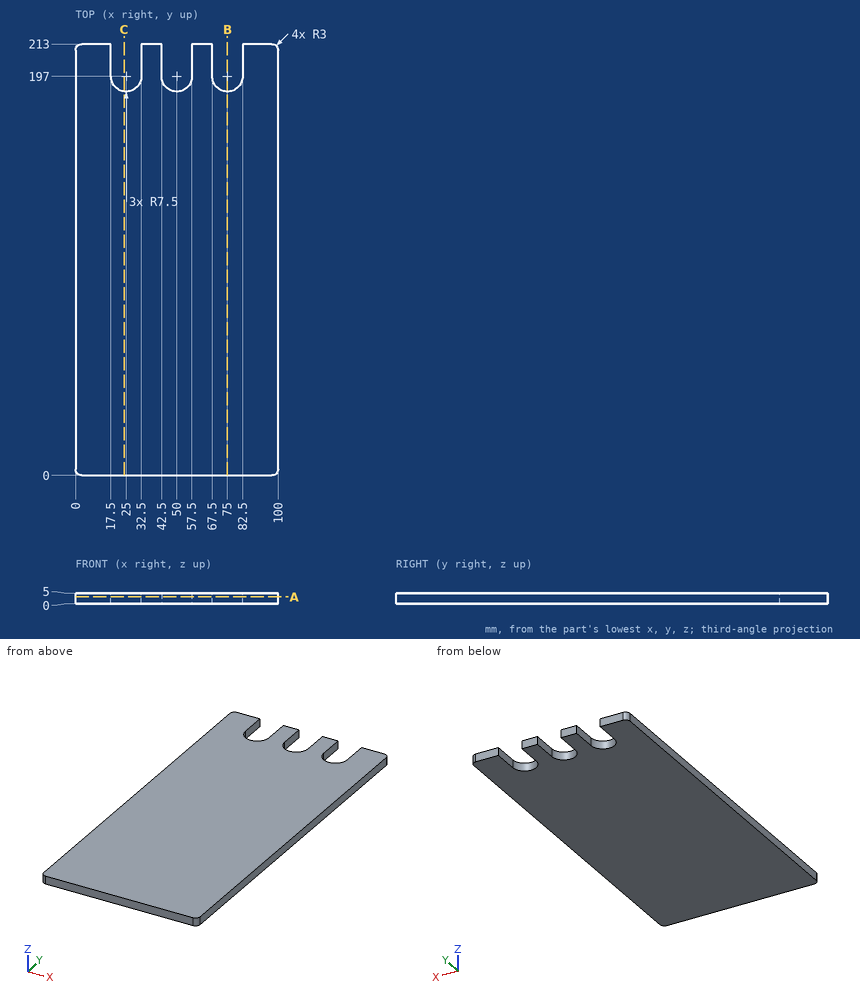
Verification items for this drawing (mm, ordinates from the low corner). Round coordinates to 2 decimals unless told otherwise and drop trailing zeros. Loops run counter-clockwise (first coordinate to the right, second up) from the corner with the lowest first, then second, coordinate; pieces in that order, holes last. Notation, with made-up numbers: (68, 72.25) - (110, 72.25) arc R24 cw to (110, 91.25) - close; hole circle Ø8 at (-20, 32). An arc over 180 degrees is marked (long way). Answer as CSV lines item,"result". Start each with the question number.
Item 1: Section check A-A (z = 3.35). Record the boundary of the cut face in (x, y).
Item 2: Scan lines: line 1 (X direction, y = 200.5, z = 3.15); line 2 (Y direction, x = 74.5, z = 2.15); line 3 (Y direction, x = 19, z = 1.8). Record each from-to range of solid material in increasing order. Write a range as [from, to].
Item 3: Section check B-B (x = 75). Record the boundary of the cut face in (y, z).
Item 4: Section check C-C (x = 24). Record the boundary of the cut face in (y, z).
Report:
1,outline,"(0, 3) arc R3 ccw to (3, 0) - (97, 0) arc R3 ccw to (100, 3) - (100, 210) arc R3 ccw to (97, 213) - (82.5, 213) - (82.5, 197) arc R7.5 cw to (67.5, 197) - (67.5, 213) - (57.5, 213) - (57.5, 197) arc R7.5 cw to (42.5, 197) - (42.5, 213) - (32.5, 213) - (32.5, 197) arc R7.5 cw to (17.5, 197) - (17.5, 213) - (3, 213) arc R3 ccw to (0, 210) - close"
2,line 1,"x = [0, 17.5], [32.5, 42.5], [57.5, 67.5], [82.5, 100]"
2,line 2,"y = [0, 189.52]"
2,line 3,"y = [0, 192.5]"
3,outline,"(0, 0) - (189.5, 0) - (189.5, 5) - (0, 5) - close"
4,outline,"(0, 0) - (189.57, 0) - (189.57, 5) - (0, 5) - close"
